Source: CAD feature listing. Evaluate the final solid. Frame: model axes, mm. A direction names the side the tool comes from. Give positions to 0.01 mm unless a question says otherwise; leave off trailing zeros. Write each loop counter-clockwise with the first axis right and the second up, starting at its lowest first coordinate (ties: lowest second). Pieces come first, ordered by that corner, then holes.
```python
from build123d import *

# Parameters (mm, degrees)
SKETCH_2_W           = 65
SKETCH_2_H           = 10
SKETCH_2_W_2         = 6
EXTRUDE_1_DEPTH      = 1
EXTRUDE_2_DEPTH      = 4
EXTRUDE_2_DEPTH_BACK = 1
SKETCH_5_W           = 15
SKETCH_5_H           = 10
SKETCH_5_W_2         = 10
SKETCH_5_H_2         = 50
EXTRUDE_3_DEPTH      = 2


with BuildPart() as part:
    # 草图2 → 凸台-拉伸1 (new body)
    with BuildSketch(Plane(origin=(0, 0, 0), x_dir=(1, 0, 0), z_dir=(0, 1, 0))):
        with Locations((-18.5, 0)):
            Rectangle(SKETCH_2_W, SKETCH_2_H)
        with Locations((-54, 0)):
            Rectangle(SKETCH_2_W_2, SKETCH_2_H)
        Polygon((-51, 15), (-61, 15), (-61, -15), (-51, -15), (-51, -5), (-57, -5), (-57, 5), (-51, 5), align=None)
        Polygon((14, 25), (14, 5), (14, -5), (14, -25), (24, -25), (24, 25), align=None)
    extrude(amount=EXTRUDE_1_DEPTH)

    # 草图4 → 凸台-拉伸2 (add, two sides)
    with BuildSketch(Plane(origin=(0, 1, 0), x_dir=(1, 0, 0), z_dir=(0, 1, 0))) as extrude_2_sk:
        Polygon((-50, -16), (-50, -6), (13, -6), (13, -26), (25, -26), (25, 26), (13, 26), (13, 6), (-50, 6), (-50, 16), (-62, 16), (-62, -16), align=None)
        Polygon((-51, -15), (-51, -5), (14, -5), (14, -25), (24, -25), (24, 25), (14, 25), (14, 5), (-51, 5), (-51, 15), (-61, 15), (-61, -15), align=None, mode=Mode.SUBTRACT)
    extrude(amount=EXTRUDE_2_DEPTH)
    extrude(extrude_2_sk.sketch, amount=-EXTRUDE_2_DEPTH_BACK)

    # 草图5 → 凸台-拉伸3 (add)
    with BuildSketch(Plane(origin=(0, 1, 0), x_dir=(1, 0, 0), z_dir=(0, 1, 0))):
        Polygon((-57, 5), (-57, -5), (-51, -5), (-51, -15), (-61, -15), (-61, 15), (-51, 15), (-51, 5), align=None)
        with Locations((-21.5, 0)):
            Rectangle(SKETCH_5_W, SKETCH_5_H)
        with Locations((19, 0)):
            Rectangle(SKETCH_5_W_2, SKETCH_5_H_2)
    extrude(amount=EXTRUDE_3_DEPTH)


solid = part.part
```
1. Section query A-A (z = 12). Return loops of the section in (x, y), plus the area to 3 significant figures.
2. Section query C-C (y = 2.2). Return loops of the section in (x, z).
3. Access query for faces 5 (the flat face through (-50, 3, 11)), 6 (the flat face through (-56, 4, 15)), 7 (the flat face through (-18, 3, -6)), 8 (the flat face through (-56, 3, -16)), 9 (the flat face through (19, 3, 26)). Directions: +Z, -Z, +X, -X, +Y, -Y. A direction counts if a zero-diameter tool reaches every point of the face in a straight line with its end or side. Return the directions, or none.
4. Pull-direction query (X, two-part tool) for faces 1 (the flat face through (-62, 3, 0)), 2 (the flat face through (14, 4, 15)), 3 (the flat face through (19, 3, 0)), 4 (the flat face through (-15, 0, 0)); classes: pulls with the +X half, pulls with the -X half, needs draft (parallel to the pull), parting line crosses it, or undercut.
5. Section query D-D (x = -26.5). Return loops of the section in (y, z), plus the area to 3 significant figures.
6. Pin query (flat end, axial travel): P1, Ø3, axis at x = -23, z = 1.5, coming from the +Y side; P2, Ø2, axis at x = -50.5, y = 2.5, coming from the -Z side; P3, Ø8, axis at x = 5.5, z = 0.5, coming from the +Y side. Return the tip coordinate at first contact, or that it passes through.
7. Line query: probe 1 along X at (y, z) = (4.4, -8); probe 2 along Z at (x, y) = (-24.5, 4.25); probe 3 along Z at (x, y) = (-52.5, 4.65). Output: solid intervals per line, ascending.
8. Section query B-B (x = -7). Return loops of the section in (y, z), plus the area to 3 significant figures.
The answers:
1. outline: (-62, 0) - (-50, 0) - (-50, 5) - (-51, 5) - (-51, 3) - (-61, 3) - (-61, 5) - (-62, 5) - close; (13, 0) - (25, 0) - (25, 5) - (24, 5) - (24, 3) - (14, 3) - (14, 5) - (13, 5) - close
1. area: 80.0 mm2
2. outline: (-62, -16) - (-50, -16) - (-50, -6) - (13, -6) - (13, -26) - (25, -26) - (25, 26) - (13, 26) - (13, 6) - (-50, 6) - (-50, 16) - (-62, 16) - close; hole (-57, -5) - (-29, -5) - (-29, 5) - (-57, 5) - close; hole (-14, -5) - (14, -5) - (14, 5) - (-14, 5) - close
3. face 5: +Z, +Y, -Y
3. face 6: +Y
3. face 7: -Z, +Y, -Y
3. face 8: -Z, -X, +Y, -Y
3. face 9: +Z, +X, -X, +Y, -Y
4. face 1: pulls with the -X half
4. face 2: undercut
4. face 3: undercut
4. face 4: needs draft
5. outline: (0, -6) - (5, -6) - (5, -5) - (3, -5) - (3, 5) - (5, 5) - (5, 6) - (0, 6) - close
5. area: 40.0 mm2
6. P1: stops at y = 3
6. P2: stops at z = -16
6. P3: stops at y = 1
7. probe 1: x = -62 to -61, -51 to -50, 13 to 14, 24 to 25
7. probe 2: z = -6 to -5, 5 to 6
7. probe 3: z = -16 to -15, 15 to 16
8. outline: (0, -6) - (5, -6) - (5, -5) - (1, -5) - (1, 5) - (5, 5) - (5, 6) - (0, 6) - close
8. area: 20.0 mm2
